Geometry: final body of the model. Coordinates: model frame, mm. Face numbers are marked on the shaded views. A direction names the side the tool comes from. Round coordinates to 2 decimals unless told otherwise and drop trailing zeros. Loops run counter-clockwise (first coordinate to the right, second up) from the corner with the lowest first, then second, coordinate; pieces in that order, holes last. Notation, with made-up numbers: (66, 55.25) -> (81, 55.25) arc R27 cw to (81, 82.25) -> close; hole circle Ø9 at (2, 58.5). An arc over 180 degrees is marked (long way). Answer in a Markdown table with one row per item.
```python
from build123d import *

# Parameters (mm, degrees)
F0_W     = 75.1286000013
F0_H     = 75.6749510765
F1_DEPTH = 25.4
F3_W     = 152.2922962904
F3_H     = 111.7689795792
F3_W_2   = 71.8111011665
F3_H_2   = 52.5860791095
F4_DEPTH = 56.896


with BuildPart() as f1:
    # F0 (on Top) → F1 (new body)
    with BuildSketch(Plane.XY):
        with Locations((37.5643000007, -37.8374755383)):
            Rectangle(F0_W, F0_H)
    extrude(amount=F1_DEPTH)


with BuildPart() as f4:
    # F3 (on Top) → F4 (new body)
    with BuildSketch(Plane.XY):
        with Locations((-0.0751465559, -0.5654413253)):
            Rectangle(F3_W, F3_H)
        with Locations((37.9036931554, -28.6490467843)):
            Rectangle(F3_W_2, F3_H_2, mode=Mode.SUBTRACT)
    extrude(amount=F4_DEPTH)


solid = f4.part
```
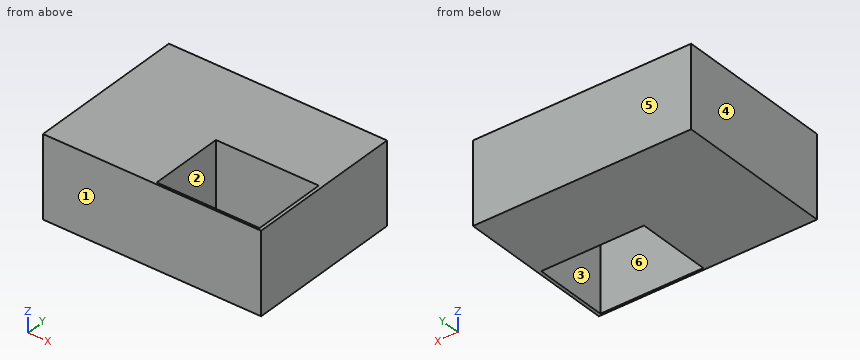
Item 1: Section query A-A, the plane x = 37. Output: boundary loops of the cut face in (y, z).
Ans:
| item | result |
|---|---|
| outline | (-56.45, 0) -> (-54.94, 0) -> (-54.94, 56.9) -> (-56.45, 56.9) -> close; (-2.36, 0) -> (55.32, 0) -> (55.32, 56.9) -> (-2.36, 56.9) -> close |
Item 2: Set-up query: the marked faces 5 and 6. Return all of +Z, -Z, +X, -X, +Y, -Y with unobstructed straight access to the full face (end or side cutting, diameter ignored); none if empty.
Ans:
| item | result |
|---|---|
| face 5 | +Z, -Z, +X, -X, +Y |
| face 6 | +Z, -Z |
Item 3: Mould query, pull axis X, two halves, no side actions, for the marked faces 1, 2, 3 and 4. Classes: released by +X, released by -X, zero draft, split by the parting line, or undercut.
Ans:
| item | result |
|---|---|
| face 1 | zero draft |
| face 2 | undercut |
| face 3 | undercut |
| face 4 | released by -X |
Item 4: Section query B-B, the plane z = 11.5. Output: boundary loops of the cut face in (x, y), and give its area (3 significant figures).
Ans:
| item | result |
|---|---|
| outline | (-76.22, -56.45) -> (76.07, -56.45) -> (76.07, 55.32) -> (-76.22, 55.32) -> close; hole (2, -54.94) -> (73.81, -54.94) -> (73.81, -2.36) -> (2, -2.36) -> close |
| area | 13,200 mm2 |
Item 5: Section query C-C, the plane y = -37.5. Output: boundary loops of the cut face in (x, z).
Ans:
| item | result |
|---|---|
| outline | (-76.22, 0) -> (2, 0) -> (2, 56.9) -> (-76.22, 56.9) -> close; (73.81, 0) -> (76.07, 0) -> (76.07, 56.9) -> (73.81, 56.9) -> close |
Item 6: Ray query, L1, parallel to Y at x = 12, z = 3; L2, parallel to X at y = -20.5, z = 19. Return the intervals inside material, ascending.
Ans:
| item | result |
|---|---|
| L1 | -56.45 to -54.94, -2.36 to 55.32 |
| L2 | -76.22 to 2, 73.81 to 76.07 |
